The listing builds one solid part. Answer for the finished solid, in the listing's coordinates (mm). A direction names the side the tool comes from. Coordinates: 2 decimals unless noted, no trailing zeros. Loops run counter-clockwise (first coordinate to the right, second up) from the corner with the lowest first, then second, coordinate; pieces in that order, holes last. Notation, with made-up numbers: (73.5, 49) - (113.5, 49) arc R23 ccw to (113.5, 61) - close; hole circle Ø2 at (77, 81). An arc over 180 degrees is marked (long way). Return JSON: item names as keys, results as strings. Group by question number.
1. The mould has two halves that part along Y. Classify faces 4 (the face through (3, 5, -10)), 5 (the face through (2, 45, -105)), 6 (the face through (5, 31, -74)): pulls with the +Y half, pulls with the -Y half, needs draft (parallel to the pull), parting line crosses it, or undercut.
2. Section D-D (x = 1.2) is taken. State how many separate pieces and enclosed holes the cut face has, and give its area (3 significant figures).
3. Find the intervals of material crossed by line 1 along Z through (x, y) = (0.65, 24.5); line 2 along Z through (x, y) = (0.45, 13); line 3 along Y through (x, z) = (1, -109), in increasing order.
4. Which of the six approach directions +Z, -Z, +X, -X, +Y, -Y give full straight-line access (tool end or side, diameter ignored) to faces 1 (the face through (2, 45, -45)), 2 (the face through (3, 8, -90)), 3 (the face through (2, 3, -60))?
5. Section C-C (z = -97) is taken. Write down the section's boundary in (x, y), and give its area (3 significant figures).
6. Section A-A (y = 26) is taken. Write down the section's boundary in (x, z).
7. This flat-tipped pin is pushed along its axis until it touches: P1, Ø2, axis at x = 4.5, y = 32, coming from the -Z side. Where does it stop, or does it pass through?
8. Section B-B (z = -67) is taken. Write down the section's boundary in (x, y), and give its area (3 significant figures).
```python
from build123d import *

# Parameters (mm, degrees)
CROQUIS1_R              = 2
SALIENTE_EXTRUIR1_DEPTH = 5
CROQUIS2_W              = 60
CROQUIS2_H              = 20
CORTAR_EXTRUIR1_DEPTH   = 10
CROQUIS3_W              = 5
CROQUIS3_H              = 40
CORTAR_EXTRUIR2_DEPTH   = 10


with BuildPart() as part:
    # Croquis1 → Saliente-Extruir1 (new body)
    with BuildSketch(Plane(origin=(0, 0, 0), x_dir=(0, 0, -1), z_dir=(1, 0, 0))):
        Polygon((0, 33.333333333), (5, 33.333333333), (5, 16.666666667), (0, 16.666666667), (0, 0), (30, 0), (30, 5), (60, 5), (60, 0), (90, 0), (90, 5), (120, 5), (120, 0), (150, 0), (150, 16.666666667), (145, 16.666666667), (145, 33.333333333), (150, 33.333333333), (150, 50), (120, 50), (120, 45), (90, 45), (90, 50), (60, 50), (60, 45), (30, 45), (30, 50), (0, 50), align=None)
        with Locations((16, 16)):
            Circle(CROQUIS1_R, mode=Mode.SUBTRACT)
        with Locations(Location((134, 16, 0), (0, 0, 180))):
            Circle(CROQUIS1_R, mode=Mode.SUBTRACT)
    extrude(amount=SALIENTE_EXTRUIR1_DEPTH)

    # Croquis2 → Cortar-Extruir1 (cut)
    with BuildSketch(Plane(origin=(5, 0, 0), x_dir=(0, 0, -1), z_dir=(1, 0, 0))):
        with Locations((90, 18)):
            Rectangle(CROQUIS2_W, CROQUIS2_H)
    extrude(amount=-CORTAR_EXTRUIR1_DEPTH, mode=Mode.SUBTRACT)

    # Croquis3 → Cortar-Extruir2 (cut)
    with BuildSketch(Plane(origin=(5, 0, 0), x_dir=(0, 0, -1), z_dir=(1, 0, 0))):
        with Locations((10.5, 25)):
            Rectangle(CROQUIS3_W, CROQUIS3_H)
    extrude(amount=-CORTAR_EXTRUIR2_DEPTH, mode=Mode.SUBTRACT)


solid = part.part
```
The answers:
{
 "1": {"face 4": "undercut", "face 5": "pulls with the +Y half", "face 6": "needs draft"},
 "2": {"separate pieces": "1", "enclosed holes": "4", "area": "5,310 mm2"},
 "3": {"line 1": "z = -145 to -120, -60 to -13, -8 to -5", "line 2": "z = -150 to -120, -60 to -13, -8 to 0", "line 3": "y = 5 to 8, 28 to 45"},
 "4": {"face 1": "+X, -X, +Y", "face 2": "+X, -X", "face 3": "+X, -X, -Y"},
 "5": {"outline": "(0, 5) - (5, 5) - (5, 8) - (0, 8) - close; (0, 28) - (5, 28) - (5, 45) - (0, 45) - close", "area": "100 mm2"},
 "6": {"outline": "(0, -145) - (5, -145) - (5, -120) - (0, -120) - close; (0, -60) - (5, -60) - (5, -13) - (0, -13) - close; (0, -8) - (5, -8) - (5, -5) - (0, -5) - close"},
 "7": {"P1": "stops at z = -145"},
 "8": {"outline": "(0, 0) - (5, 0) - (5, 8) - (0, 8) - close; (0, 28) - (5, 28) - (5, 50) - (0, 50) - close", "area": "150 mm2"}
}
